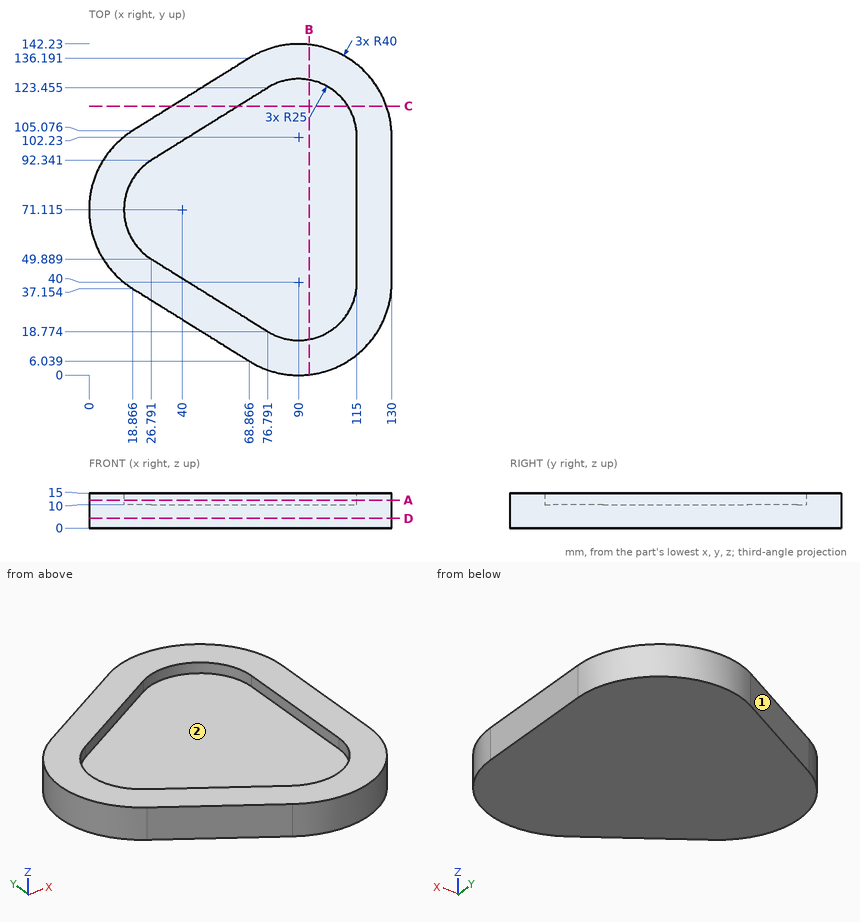
Design review of the part shown in the three views and the two pictorial views. Dimensions are in mm from the part's minimum x, y and z. A direction names the side the tool comes from. Round coordinates to 2 decimals unless told otherwise and drop trailing zeros. Loops run counter-clockwise (first coordinate to the right, second up) from the corner with the lowest first, then second, coordinate; pieces in that order, holes last.
Q1. Insertion check: pin 1 Ø5 at (x, z) = (65, 12.5) entering from +Y; pin 2 Ø5 at (x, z) = (75.5, 7.5) entering from -Y; pin 3 Ø6 at (y, z) = (126.5, 5.5) entering from -X (1 decimal). Each pin has a flat end and moves straight along its axis. Give the tip position at first contact, or say it passes through.
Result sheet:
pin 1: stops at y = 135.34
pin 2: stops at y = 1.84
pin 3: stops at x = 48.5
Q2. Add section B-B on x = 94.5. Write out the cut boundary in (y, z) (1 decimal), plus the area to 3 significant figures.
Result sheet:
outline: (0.3, 0) - (142, 0) - (142, 15) - (126.8, 15) - (126.8, 10) - (15.4, 10) - (15.4, 15) - (0.3, 15) - close
area: 1,570 mm2
Q3. Add section A-A on z = 12. Write out the cut boundary in (x, y) (1 decimal).
Result sheet:
outline: (18.9, 37.2) - (68.9, 6) arc R40 ccw to (130, 40) - (130, 102.2) arc R40 ccw to (68.9, 136.2) - (18.9, 105.1) arc R40 ccw to start; hole (26.8, 49.9) - (76.8, 18.8) arc R25 ccw to (115, 40) - (115, 102.2) arc R25 ccw to (76.8, 123.5) - (26.8, 92.3) arc R25 ccw to start
Q4. Add section C-C on y = 115.5. Write out the cut boundary in (x, z) (1 decimal).
Result sheet:
outline: (35.6, 0) - (127.7, 0) - (127.7, 15) - (111.2, 15) - (111.2, 10) - (64, 10) - (64, 15) - (35.6, 15) - close
Q5. Machinability: for the marked faces 1 and 2, which of the approach directions +Z, -Z, +X, -X, +Y, -Y give a long, thin tool a straight path to every point of the face, cutting with its end or side? Answer none if there is none.
Result sheet:
face 1: +Z, -Z, -X, +Y
face 2: +Z
Q6. Add section D-D on z = 4.25. Write out the cut boundary in (x, y) (1 decimal), plus the area to 3 significant figures.
Result sheet:
outline: (18.9, 37.2) - (68.9, 6) arc R40 ccw to (130, 40) - (130, 102.2) arc R40 ccw to (68.9, 136.2) - (18.9, 105.1) arc R40 ccw to start
area: 13,800 mm2
Q7. To check wall thickness, follow line 1 along Z through (x, y) = (26.5, 78); line 2 along Y through (x, z) = (77, 12.5) (1 decimal); line 3 along Y through (x, z) = (85, 12) (1 decimal). State the ranges of each line that lie inside material, in increasing order.
Result sheet:
line 1: z = 0 to 10
line 2: y = 2.2 to 18.6, 123.6 to 140.1
line 3: y = 0.3 to 15.5, 126.7 to 141.9
